Check sheet for the drawn part. Datum: minimum x, y, z corner. Units: mm. A direction names the side the tool comes from. Coordinates: 2 decimals unless noted, no trailing zeros. Loops run counter-clockwise (first coordinate to the right, second up) from the corner with the lowest first, then second, coordinate; pieces in that order, holes last. Notation, with made-up numbers: (-20.5, -36) - (30.5, -36) arc R9 cw to (30.5, -19) - close; hole circle Ø2 at (-12.75, 17). An arc over 180 degrees is marked (long way). Write item = value, one per line. Start each with the question number.
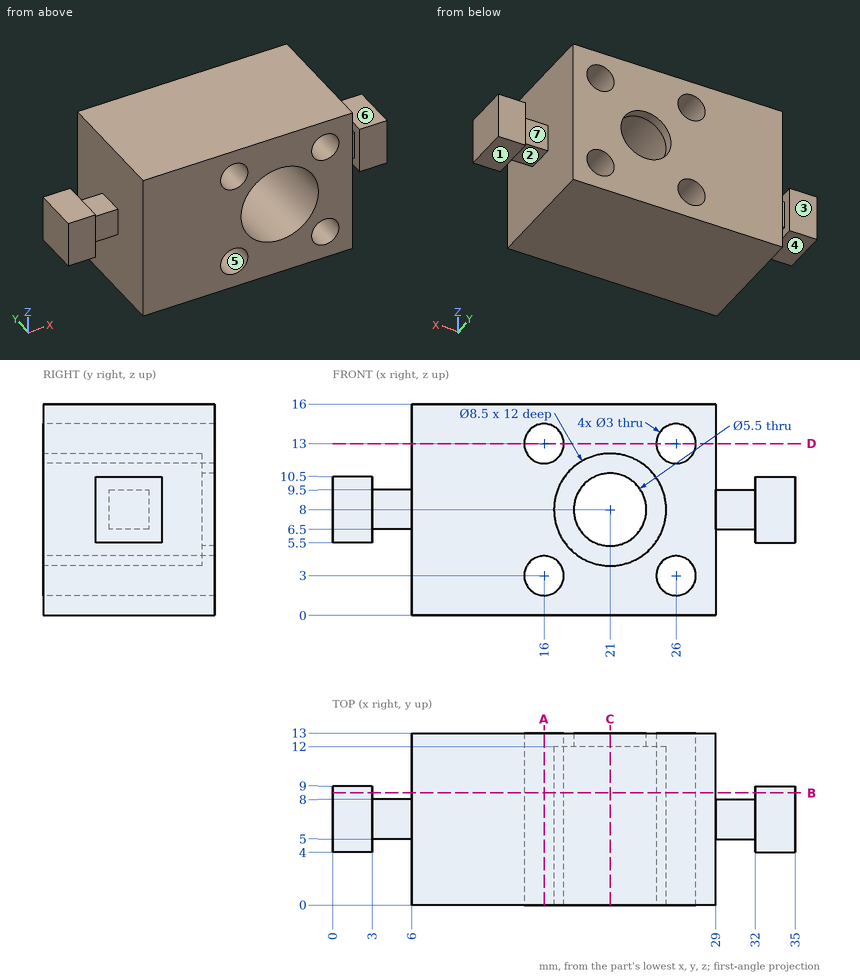
(1) Sectioned sample at C-C on x = 21. Enter the section's corners in (y, z), plus the area to 4 significant figures.
(2) Tool access check on the marked faces 1, 2, 3 and 4. Record the directions out of +Z, -Z, +X, -X, +Y, -Y that give a thin tool (end or side, any length) a straight path to the whole face; none if there is none.
(3) Sectioned sample at A-A on x = 16. Enter the section's corners in (y, z).
(4) Sectioned sample at D-D on z = 13. Enter the section's corners in (x, y).
(5) Scan lines: line 1 (Z direction, x = 26, y = 6.25); line 2 (Z direction, x = 21, y = 6.5); line 3 (X direction, y = 8.5, z = 8.25). Record each from-to range of solid material in increasing order.
(6) Sectioned sample at B-B on y = 8.5. Enter the section's corners in (x, z).
(7) Draft check along Z on the marked faces 5, 6 and 7. Enter one of: pulls with the +Z half, pulls with the -Z half, needs draft (parallel to the pull), parting line crosses it, or undercut.
(8) Depth check by flat-ended pin: pin 1 (3.5 mm diameter, centred on x = 33, y = 7, fed in from -Z); pin 2 (3.5 mm diameter, centred on x = 33.5, z = 8.5, fed in from -Y); pin 3 (2 mm diameter, centred on y = 2.5, z = 8.5, fed in from -X); pin 4 (2.5 mm diameter, centred on x = 16, z = 3, fed in from +Y). Enter the tip coordinate at first touch or a pass-through.
Working result:
q1.outline = (0, 0) - (13, 0) - (13, 5.25) - (12, 5.25) - (12, 3.75) - (0, 3.75) - close; (0, 12.25) - (12, 12.25) - (12, 10.75) - (13, 10.75) - (13, 16) - (0, 16) - close
q1.area = 100.5 mm2
q2.face_1 = -Z, +X, +Y, -Y
q2.face_2 = -Z, +Y, -Y
q2.face_3 = +Z, -Z, -X, +Y
q2.face_4 = -Z, -X, +Y, -Y
q3.outline = (0, 0) - (13, 0) - (13, 1.5) - (0, 1.5) - close; (0, 4.5) - (13, 4.5) - (13, 11.5) - (0, 11.5) - close; (0, 14.5) - (13, 14.5) - (13, 16) - (0, 16) - close
q4.outline = (6, 0) - (14.5, 0) - (14.5, 13) - (6, 13) - close; (17.5, 0) - (24.5, 0) - (24.5, 13) - (17.5, 13) - close; (27.5, 0) - (29, 0) - (29, 13) - (27.5, 13) - close
q5.line_1 = 0 to 1.5, 4.5 to 11.5, 14.5 to 16
q5.line_2 = 0 to 3.75, 12.25 to 16
q5.line_3 = 0 to 3, 6 to 16.76, 25.24 to 29, 32 to 35
q6.outline = (0, 5.5) - (3, 5.5) - (3, 10.5) - (0, 10.5) - close; (6, 0) - (29, 0) - (29, 16) - (6, 16) - close; (32, 5.5) - (35, 5.5) - (35, 10.5) - (32, 10.5) - close; hole circle Ø3 at (16, 3); hole circle Ø3 at (16, 13); hole circle Ø8.5 at (21, 8); hole circle Ø3 at (26, 3); hole circle Ø3 at (26, 13)
q7.face_5 = undercut
q7.face_6 = pulls with the +Z half
q7.face_7 = needs draft
q8.pin_1 = 5.5
q8.pin_2 = 4
q8.pin_3 = 6
q8.pin_4 = through
